The model under review builds one solid part; all positions refer to its coordinate system, in mm. Face numbers are marked on the shaded views. A direction names the side the tool comes from. Coordinates: 2 decimals unless noted, no trailing zeros. Write each loop counter-clockwise with the first axis right and the second up, starting at its lowest first coordinate (ties: lowest second). Pieces come first, ordered by that corner, then holes.
1) Add section B-B, the plane x = -970. State the section outline as (y, z) points, then the cut area to 3 significant figures.
2) Add section D-D, the plane y = -176. State the section outline as (x, z) points.
3) Machinability: for the marked faces 1 and 2, which of the approach directions +Z, -Z, +X, -X, +Y, -Y give a long, thin tool a straight path to every point of the face, cutting with its end or side? Answer none if there is none.
4) For P1, Ø8, axis at x = -1010, z = 103.5, coming from the -Y side; P2, Ø18.5, axis at y = -180.5, z = 153, coming from the -X side; P3, Ø12, axis at y = -204.5, z = 287, coming from the +X side; P4, Ø1, axis at x = -995, y = -188, coming from the +Z side, all flat-tipped, find the tip position at first contact; note any pin that passes through.
5) Add section C-C, the plane y = -144.5. State the section outline as (x, z) points, then the cut area to 3 significant figures.
6) Add section A-A, the plane z = 372. State the section outline as (x, y) points, then the cut area to 3 significant figures.
7) For line 1 (Y direction, x = -997.5, z = 65.5); line 2 (Y direction, x = -1003.5, z = 342); line 3 (X direction, y = -168.5, z = 132), list the stretches that pass through material, from the lowest coordinate up.
from build123d import *

# Parameters (mm, degrees)
SKETCH004_W   = 100
SKETCH004_H   = 100
PAD002_DEPTH  = 2
SKETCH005_W   = 40
SKETCH005_H   = 40
SKETCH005_W_2 = 37
SKETCH005_H_2 = 37
PAD003_DEPTH  = 458
SKETCH006_W   = 100
SKETCH006_H   = 100
SKETCH006_W_2 = 97
SKETCH006_H_2 = 97
PAD004_DEPTH  = 100


with BuildPart() as part:
    # Sketch004 → Pad002 (new body)
    with BuildSketch(Plane.XY):
        with Locations((-1000, -180)):
            Rectangle(SKETCH004_W, SKETCH004_H)
    extrude(amount=PAD002_DEPTH)

    # Sketch005 (on Face6 of Pad002) → Pad003 (join)
    with BuildSketch(Plane.XY.offset(2)):
        with Locations((-1000, -180)):
            Rectangle(SKETCH005_W, SKETCH005_H)
        with Locations((-1000, -180)):
            Rectangle(SKETCH005_W_2, SKETCH005_H_2, mode=Mode.SUBTRACT)
    extrude(amount=PAD003_DEPTH)

    # Sketch006 → Pad004 (join)
    with BuildSketch(Plane.XY):
        with Locations((-1000, -180)):
            Rectangle(SKETCH006_W, SKETCH006_H)
        with Locations((-1000, -180)):
            Rectangle(SKETCH006_W_2, SKETCH006_H_2, mode=Mode.SUBTRACT)
    extrude(amount=PAD004_DEPTH)


solid = part.part
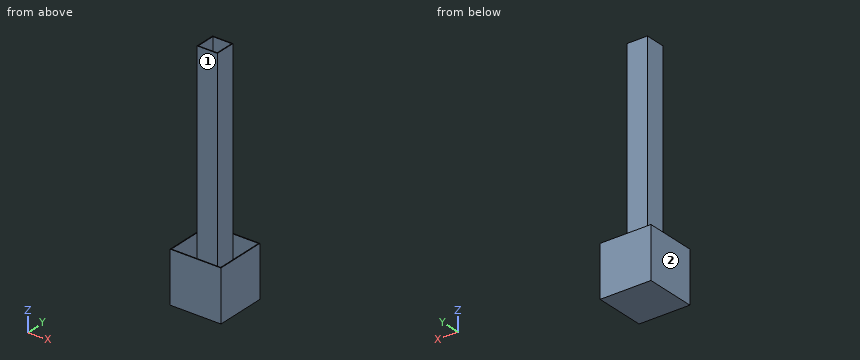
Geometry results:
1. outline: (-230, 0) - (-130, 0) - (-130, 100) - (-131.5, 100) - (-131.5, 2) - (-228.5, 2) - (-228.5, 100) - (-230, 100) - close
1. area: 494 mm2
2. outline: (-1050, 0) - (-950, 0) - (-950, 100) - (-951.5, 100) - (-951.5, 2) - (-980, 2) - (-980, 460) - (-981.5, 460) - (-981.5, 2) - (-1018.5, 2) - (-1018.5, 460) - (-1020, 460) - (-1020, 2) - (-1048.5, 2) - (-1048.5, 100) - (-1050, 100) - close
3. face 1: +Z
3. face 2: +Z, -Z, -X, +Y, -Y
4. P1: stops at y = -230
4. P2: stops at x = -1020
4. P3: stops at x = -980
4. P4: stops at z = 2
5. outline: (-1050, 0) - (-950, 0) - (-950, 100) - (-951.5, 100) - (-951.5, 2) - (-1048.5, 2) - (-1048.5, 100) - (-1050, 100) - close
5. area: 494 mm2
6. outline: (-1020, -200) - (-980, -200) - (-980, -160) - (-1020, -160) - close; hole (-1018.5, -198.5) - (-981.5, -198.5) - (-981.5, -161.5) - (-1018.5, -161.5) - close
6. area: 231 mm2
7. line 1: y = -230 to -228.5, -200 to -198.5, -161.5 to -160, -131.5 to -130
7. line 2: y = -200 to -198.5, -161.5 to -160
7. line 3: x = -1020 to -1018.5, -981.5 to -980
